Part model, mm, in its own coordinate system. A direction names the side the tool comes from. Round coordinates to 2 decimals unless told otherwise and drop trailing zeros. Order: outer loops, then holes, each group sorted by start corner. A loop starts at its lowest first (then second) coordinate and runs counter-clockwise, first axis right, second up. Notation, with made-up numbers: (89, -25) - (122, -25) arc R18 cw to (122, -8) - close; hole circle Ø8 at (20.25, 56.5). An arc over 180 degrees is marked (long way). Answer as a JSON object with one key per item and string values.
```python
from build123d import *

# Parameters (mm, degrees)
BOSS_EXTRUDE1_DEPTH      = 74.93
BOSS_EXTRUDE4_DEPTH      = 2.54
BOSS_EXTRUDE4_DEPTH_BACK = 2.54
BOSS_EXTRUDE6_DEPTH      = 74.93
BOSS_EXTRUDE7_DEPTH      = 74.93
SKETCH11_R               = 3.3782
BOSS_EXTRUDE8_DEPTH      = 2.54
SKETCH13_R               = 3.971263101
BOSS_EXTRUDE10_DEPTH     = 5.08
SKETCH12_R               = 3.175
BOSS_EXTRUDE9_DEPTH      = 5.08


with BuildPart() as part:
    # Sketch1 → Boss-Extrude1 (new body)
    with BuildSketch(Plane.XY):
        with BuildLine():
            Line((-16.295773791, 0.624640473), (-12.907508233, 0.624640473))
            Line((-12.907508233, 0.624640473), (-12.443267089, 3.164640473))
            add(Edge.make_bspline(
                [(-12.443267089, 3.164640473), (-12.30668745, 3.911907895), (-11.89696139, 6.153716378), (-11.35075536, 9.142778811), (-10.941162808, 11.384616955), (-10.804635025, 12.131895145)],
                knots=[0.002076118, 0.002076118, 0.002076118, 0.002076118, 0.004355051, 0.008912916, 0.011191849, 0.011191849, 0.011191849, 0.011191849], degree=3))
            add(Edge.make_bspline(
                [(-10.804635025, 12.131895145), (-10.131787944, 14.813925559), (-8.428636773, 20.08894476), (-4.769918918, 27.602373316), (-0.882056925, 33.370017928), (2.696640916, 37.629074894), (4.663596703, 39.6688962), (5.677623009, 40.647244333)],
                knots=[-0.595137067, -0.595137067, -0.595137067, -0.595137067, -0.254899084, 0.0853389, 0.425576884, 0.595695875, 0.765814867, 0.765814867, 0.765814867, 0.765814867], degree=3))
            Line((5.677623009, 40.647244333), (2.03170084, 44.371046934))
            add(Edge.make_bspline(
                [(2.03170084, 44.371046934), (1.545061943, 43.849333503), (0.584048879, 42.784657511), (-1.227882281, 40.634272171), (-4.205920413, 36.737641226), (-7.868630072, 30.842728735), (-11.285075765, 23.259160615), (-12.891126954, 17.928422411), (-13.516382283, 15.22778531)],
                knots=[0.192222826, 0.192222826, 0.192222826, 0.192222826, 0.287167093, 0.38211136, 0.571999893, 0.951776961, 1.331554028, 1.711331096, 1.711331096, 1.711331096, 1.711331096], degree=3))
            add(Edge.make_bspline(
                [(-13.516382283, 15.22778531), (-13.707651088, 14.222513225), (-14.09021448, 12.211975656), (-14.664139503, 9.196174334), (-15.238140346, 6.180406911), (-15.620861993, 4.169893716), (-15.812232602, 3.164640473)],
                knots=[-0.00268258, -0.00268258, -0.00268258, -0.00268258, 0.000387339, 0.003457258, 0.006527177, 0.009597097, 0.009597097, 0.009597097, 0.009597097], degree=3))
            Line((-15.812232602, 3.164640473), (-16.295773791, 0.624640473))
        make_face()
    extrude(amount=BOSS_EXTRUDE1_DEPTH)

    # Sketch4 → Boss-Extrude4 (add, two sides: drawn at the far end of the back side and taken through both)
    with BuildSketch(Plane(origin=(0, 0, 37.465), x_dir=(-1, 0, 0), z_dir=(0, 0, -1)).offset(-BOSS_EXTRUDE4_DEPTH_BACK)):
        with BuildLine():
            Line((-5.677623009, 40.647244333), (-2.087143894, 44.314419562))
            ThreePointArc((-2.087143894, 44.314419562), (-5.945357936, 46.761917563), (-10.144870483, 48.561961011))
            Line((-10.144870483, 48.561961011), (-12.342217859, 43.933321468))
            ThreePointArc((-12.342217859, 43.933321468), (-8.878894593, 42.556020468), (-5.677623009, 40.647244333))
        make_face()
    extrude(amount=BOSS_EXTRUDE4_DEPTH + BOSS_EXTRUDE4_DEPTH_BACK)

    # Sketch8 → Boss-Extrude6 (add)
    with BuildSketch(Plane(origin=(0, 0, 0), x_dir=(-1, 0, 0), z_dir=(0, 0, -1))):
        with BuildLine():
            Line((12.199993526, 0.628671187), (16.843743367, 0.628671187))
            add(Edge.make_bspline(
                [(-2.03170084, 44.371046934), (15.008940659, 25.494574417), (16.843743367, 0.628671187)],
                knots=[0, 0, 0, 1, 1, 1], degree=2))
            Line((-2.03170084, 44.371046934), (-5.677623009, 40.647244333))
            add(Edge.make_bspline(
                [(-5.677623009, 40.647244333), (9.879032096, 23.52153238), (12.199993526, 0.628671187)],
                knots=[0, 0, 0, 1, 1, 1], degree=2))
        make_face()
    extrude(amount=-BOSS_EXTRUDE6_DEPTH)

    # Sketch10 → Boss-Extrude7 (add)
    with BuildSketch(Plane.XY.offset(74.93)):
        with BuildLine():
            add(Edge.make_bspline(
                [(-17.044210577, -3.569022053), (-16.99706974, -1.449262713), (-16.843743367, 0.628671187)],
                knots=[0, 0, 0, 1, 1, 1], degree=2))
            Line((-16.843743367, 0.628671187), (-16.295006462, 0.628671187))
            Line((-16.295006462, 0.628671187), (-16.295773791, 0.624640473))
            Line((-16.295773791, 0.624640473), (-12.907508233, 0.624640473))
            Line((-12.907508233, 0.624640473), (-12.906771531, 0.628671187))
            Line((-12.906771531, 0.628671187), (-12.199993526, 0.628671187))
            add(Edge.make_bspline(
                [(-12.199993526, 0.628671187), (-12.410380076, -1.44648182), (-12.512012235, -3.569022053)],
                knots=[0, 0, 0, 1, 1, 1], degree=2))
            Line((-12.512012235, -3.569022053), (-17.044210577, -3.569022053))
        make_face()
    extrude(amount=-BOSS_EXTRUDE7_DEPTH)

    # Sketch11 → Boss-Extrude8 (add, symmetric)
    with BuildSketch(Plane(origin=(0, 0, 37.465), x_dir=(-1, 0, 0), z_dir=(0, 0, -1))):
        with BuildLine():
            Line((-6.661684739, 45.739942581), (-10.144870483, 48.561961011))
            Line((-10.144870483, 48.561961011), (-21.30072948, 34.383167777))
            ThreePointArc((-21.30072948, 34.383167777), (-21.992768178, 32.976186787), (-22.052439991, 31.409358033))
            add(Edge.make_bspline(
                [(-43.921175132, 3.682891736), (-14.804010115, 3.685410597), (-22.052439991, 31.409358033)],
                knots=[0, 0, 0, 1, 1, 1], degree=2))
            ThreePointArc((-43.921175132, 3.682891736), (-45.398270297, 3.247037241), (-46.577742371, 2.256772178))
            Line((-46.577742371, 2.256772178), (-48.989981542, -0.809118172))
            ThreePointArc((-48.989981542, -0.809118172), (-49.700911454, -0.673916534), (-50.423765203, -0.639517698))
            Line((-50.423765203, -0.639517698), (-54.431438085, 15.399576445))
            ThreePointArc((-54.431438085, 15.399576445), (-57.076455171, 16.988173168), (-58.666731899, 14.344165819))
            Line((-58.666731899, 14.344165819), (-54.431438085, -2.697927839))
            ThreePointArc((-54.431438085, -2.697927839), (-50.902490469, -10.922372789), (-45.581657306, -3.726283541))
            Line((-45.581657306, -3.726283541), (-43.706337234, -1.342802757))
            ThreePointArc((-43.706337234, -1.342802757), (-42.430425985, -0.374532318), (-40.844196848, -0.152329073))
            ThreePointArc((-40.844196848, -0.152329073), (-20.926969962, 8.132007566), (-17.561546975, 29.439285396))
            ThreePointArc((-17.561546975, 29.439285396), (-17.718806517, 31.033263625), (-17.077929798, 32.501178536))
            Line((-17.077929798, 32.501178536), (-11.948808892, 39.020151644))
            Line((-11.948808892, 39.020151644), (-6.661684739, 45.739942581))
        make_face()
        with Locations((-50.306976812, -5.797526095)):
            Circle(SKETCH11_R, mode=Mode.SUBTRACT)
    extrude(amount=BOSS_EXTRUDE8_DEPTH, both=True)

    # Sketch13 → Boss-Extrude10 (add)
    with BuildSketch(Plane.XY.offset(40.005)):
        with Locations((56.548749752, 14.870525834)):
            Circle(SKETCH13_R)
    extrude(amount=-BOSS_EXTRUDE10_DEPTH)

    # Sketch12 → Boss-Extrude9 (add)
    with BuildSketch(Plane.XY.offset(40.005)):
        with Locations(Location((56.548749752, 14.870525834, 0), (0, 0, 180))):
            Circle(SKETCH12_R)
    extrude(amount=BOSS_EXTRUDE9_DEPTH)


solid = part.part
```
Item 1: Probe L1, parallel to Z at x = 45.5, y = 3 (3 decimals); L2, parallel to X at y = 28.5, z = 35 (3 decimals); L3, parallel to Y at x = 45, z = 36. List the from-to ranges inside material, lowest first. Write a range as from..to.
Taken from the geometry:
{"L1": "34.925..40.005", "L2": "-9.07..-3.275, 17.239..21.376", "L3": "-2.99..3.43"}
Item 2: Two-plate mould, pull along X, no slides. Class faces 5 (the flat face through (-8, 22, 0)), 6 (the flat face through (47.767, 0.745, 37.429)), 7 (the cylindrical face through (51.053, -10.903, 37.429)): pulls with the +X half, pulls with the -X half, needs draft (parallel to the pull), parting line crosses it, or undercut.
Taken from the geometry:
{"face 5": "needs draft", "face 6": "undercut", "face 7": "parting line crosses it"}
Item 3: Cut at B-B (x = 8). Write the cut outline in (y, z) (3 decimals).
Taken from the geometry:
{"outline": "(42.099, 34.925) - (47.742, 34.925) - (47.742, 40.005) - (42.099, 40.005) - close"}
Item 4: Drop flat-ended pins along their axis: P1, Ø1.9, axis at x = 57, y = 16.5, coming from the +Z side (3 decimals); P2, Ø4, axis at x = 19.5, y = 36.5, coming from the -Z side (3 decimals); P3, Ø10, axis at y = -2.5, z = 33.5, coming from the +X side. Give the stop position or say it passes through.
Taken from the geometry:
{"P1": "z = 45.085", "P2": "z = 34.925", "P3": "x = 55.67"}
Item 5: Cut at A-A (y = -7). Write the cut outline in (x, z) (3 decimals).
Taken from the geometry:
{"outline": "(45.29, 34.925) - (47.15, 34.925) - (47.15, 40.005) - (45.29, 40.005) - close; (53.464, 34.925) - (55.324, 34.925) - (55.324, 40.005) - (53.464, 40.005) - close"}
Item 6: Tool access for faces 1 (the cylindrical face through (45.379, 3.257, 37.429)), 2 (the flat face through (44.657, -2.551, 37.429)), 3 (the cylindrical face through (7.364, 41.738, 37.501)), 4 (the flat face through (57, 15, 45.085)): list every direction of +Z, -Z, +X, -X, +Y, -Y with a clear straight run to the whole face (end or side of a thin tool).
Taken from the geometry:
{"face 1": "+Z, -Z, +Y", "face 2": "+Z, -Z", "face 3": "+Z, -Z, -Y", "face 4": "+Z, +X, +Y, -Y"}
